from build123d import *

# Parameters (mm, degrees)
SKETCH1_R           = 3.399999992
SKETCH1_R_2         = 4.999999996
SKETCH1_R_3         = 3.4
SKETCH1_R_4         = 2.499999993
SKETCH1_R_5         = 3.399999999
SKETCH1_R_6         = 3.5
SKETCH1_R_7         = 4.999999995
SKETCH1_R_8         = 2.5
SKETCH1_R_9         = 3.999999996
BOSS_EXTRUDE1_DEPTH = 3


with BuildPart() as part:
    # Sketch1 → Boss-Extrude1 (new body)
    with BuildSketch(Plane.XY):
        with BuildLine():
            Line((-376.085243079, -163.278565422), (-350.152013506, -163.278565422))
            Line((-350.152013506, -163.278565422), (-20.152013506, -163.278565422))
            Line((-20.152013506, -163.278565422), (56.677553307, -117.080446425))
            ThreePointArc((56.677553307, -117.080446425), (63.779903671, -109.786095566), (66.371177049, -99.940475351))
            Line((66.371177049, -99.940475351), (66.371177049, 7.470187014))
            ThreePointArc((66.371177049, 7.470187014), (60.513312673, 21.612322638), (46.371177049, 27.470187014))
            Line((46.371177049, 27.470187014), (-56.693059514, 27.470187014))
            ThreePointArc((-56.693059514, 27.470187014), (-58.857455653, 27.707226943), (-60.919242131, 28.407109144))
            Line((-60.919242131, 28.407109144), (-362.409808619, 168.994469159))
            ThreePointArc((-362.409808619, 168.994469159), (-370.173396171, 169.284827359), (-375.801891017, 163.92967607))
            ThreePointArc((-375.801891017, 163.92967607), (-409.999846255, 0.355046993), (-376.085243079, -163.278565422))
        make_face()
        with Locations((-367.783184481, -144.245762074)):
            Circle(SKETCH1_R, mode=Mode.SUBTRACT)
        with Locations((-373.28475698, -129.22135859)):
            Circle(SKETCH1_R_2, mode=Mode.SUBTRACT)
        with Locations((-378.786329478, -114.196955106)):
            Circle(SKETCH1_R_3, mode=Mode.SUBTRACT)
        with Locations((-260.152013506, -143.278565422)):
            Circle(SKETCH1_R_4, mode=Mode.SUBTRACT)
        with Locations((-200.152013506, -143.278565422)):
            Circle(SKETCH1_R_4, mode=Mode.SUBTRACT)
        with Locations((-400.403512963, -3.404677757)):
            Circle(SKETCH1_R_5, mode=Mode.SUBTRACT)
        with BuildLine():
            ThreePointArc((-278.689644498, -129.955115483), (-307.207328121, -13.412961613), (-288.955480876, 105.171194074))
            Line((-288.955480876, 105.171194074), (-254.820961391, 89.254006231))
            ThreePointArc((-254.820961391, 89.254006231), (-269.078930784, -22.282930678), (-236.667843088, -129.955115483))
            Line((-236.667843088, -129.955115483), (-278.689644498, -129.955115483))
        make_face(mode=Mode.SUBTRACT)
        with Locations((-140.152013506, -143.278565422)):
            Circle(SKETCH1_R_4, mode=Mode.SUBTRACT)
        with Locations((-80.152013506, -143.278565422)):
            Circle(SKETCH1_R_4, mode=Mode.SUBTRACT)
        with Locations((-24, 0)):
            Circle(SKETCH1_R_6, mode=Mode.SUBTRACT)
        with BuildLine():
            ThreePointArc((5.00000001, 2e-09), (-1.082198053, -4.881480028), (-4.531538915, 2.113091308))
            ThreePointArc((-4.531538915, 2.113091308), (1.082198084, 4.881480032), (5.00000001, 2e-09))
        make_face(mode=Mode.SUBTRACT)
        with Locations((24, 0)):
            Circle(SKETCH1_R_6, mode=Mode.SUBTRACT)
        with Locations((-399.802415875, 12.570928686)):
            Circle(SKETCH1_R_7, mode=Mode.SUBTRACT)
        with Locations((-399.154276158, 28.570928686)):
            Circle(SKETCH1_R_3, mode=Mode.SUBTRACT)
        with BuildLine():
            ThreePointArc((-316.911336344, 115.346293338), (-337.157938663, 7.879523189), (-321.95378618, -100.415746047))
            ThreePointArc((-321.95378618, -100.415746047), (-325.402488065, -106.990809188), (-331.977551206, -103.542107303))
            ThreePointArc((-331.977551206, -103.542107303), (-347.65507241, 8.124845631), (-326.778108863, 118.937504843))
            ThreePointArc((-326.77810886, 118.937504842), (-320.933069671, 122.312139792), (-316.594722606, 117.141899091))
            ThreePointArc((-316.594722606, 117.141899091), (-316.674481903, 116.230246159), (-316.911336347, 115.346293339))
        make_face(mode=Mode.SUBTRACT)
        with Locations((-384.276933996, 115.256858232)):
            Circle(SKETCH1_R_8, mode=Mode.SUBTRACT)
        with Locations((-333.868117351, 124.060751978)):
            Circle(SKETCH1_R_8, mode=Mode.SUBTRACT)
        with Locations((-304.866268166, 110.536967602)):
            Circle(SKETCH1_R_8, mode=Mode.SUBTRACT)
        with Locations((-377.386541732, 132.587322578)):
            Circle(SKETCH1_R_9, mode=Mode.SUBTRACT)
        with Locations((-370.496149468, 149.917786924)):
            Circle(SKETCH1_R_8, mode=Mode.SUBTRACT)
    extrude(amount=BOSS_EXTRUDE1_DEPTH)


solid = part.part
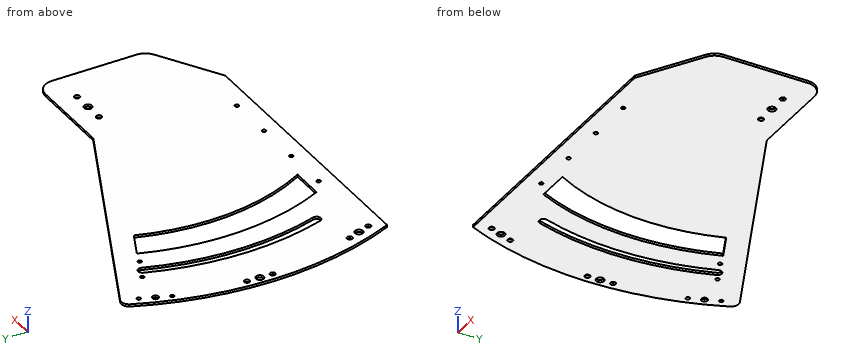
The listing builds one solid part. Answer for the finished solid, in the listing's coordinates (mm). Coordinates: 2 decimals unless noted, no trailing zeros. Loops run counter-clockwise (first coordinate to the right, second up) from the corner with the lowest first, then second, coordinate; pieces in that order, holes last. Notation, with made-up numbers: (17, -27) -> (35, -27) arc R22 ccw to (35, 2) -> close; hole circle Ø6 at (6.5, 38). An arc over 180 degrees is marked (long way). Answer in a Markdown table with one row per item. Add a question column.
1. The part is cut by section A-A, the plane y = 46.5. Write down the section's boundary in (x, z).
2. The part is cut by section D-D, the plane x = -96.5. Write down the section's boundary in (y, z), then the cut area to 3 significant figures.
3. The part is cut by section B-B, the plane x = -218. Write down the section's boundary in (y, z).
4. Flat-ended cylindrical pins translate along their axes: P1, Ø4, axis at x = 24, y = 0, coming from the -Z side; P2, Ø0.9, axis at x = -250, z = 1.5, coming from the +Y side; P3, Ø1.5, axis at x = -18, z = 1.5, coming from the +Y side. Find the tip coordinate at first contact, or state that the pin passes through.
5. The part is cut by section C-C, the plane z = 1.75. Count the separate pieces of the cut face and the enclosed holes in it, then the cut area to 3 significant figures.
6. Consider line 1 (X direction, y = 116, z = 2.55); line 2 (X direction, y = -36.5, z = 1.45); line 3 (X direction, y = 8, z = 0.35). Determine where each line is inside the solid, lowest interval first. Write a range as [from, to].
Answer below:
| question | item | result |
|---|---|---|
| 1 | outline | (-407.35, 0) -> (-344.63, 0) -> (-344.63, 3) -> (-407.35, 3) -> close; (-334.03, 0) -> (-303.96, 0) -> (-303.96, 3) -> (-334.03, 3) -> close; (-265.97, 0) -> (-99.72, 0) -> (-99.72, 3) -> (-265.97, 3) -> close |
| 2 | outline | (-163.28, 0) -> (45, 0) -> (45, 3) -> (-163.28, 3) -> close |
| 2 | area | 625 mm2 |
| 3 | outline | (-163.28, 0) -> (101.66, 0) -> (101.66, 3) -> (-163.28, 3) -> close |
| 4 | P1 | through |
| 4 | P2 | y = 116.79 |
| 4 | P3 | y = 27.47 |
| 5 | separate pieces | 1 |
| 5 | enclosed holes | 20 |
| 5 | area | 101,000 mm2 |
| 6 | line 1 | [-393.25, -386.66], [-381.89, -327.83], [-316.72, -248.76] |
| 6 | line 2 | [-408.37, -345.83], [-335.27, -305.33], [-267.52, 66.37] |
| 6 | line 3 | [-409.92, -401.83], [-397.78, -347.66], [-337.16, -307.4], [-269.88, 66.36] |
